from build123d import *

# Parameters (mm, degrees)
BOSS_EXTRUDE1_START         = -123.825
BOSS_EXTRUDE1_OUTLINE_R     = 6.35
BOSS_EXTRUDE1_DEPTH         = 130.175
SKETCH5_W                   = 1.4224
SKETCH5_H                   = 0.4064
F_1_4_20_TAPPED_HOLE1_D     = 5.1054
F_1_4_20_TAPPED_HOLE1_DEPTH = 16.51
F_1_4_20_TAPPED_HOLE1_TIP   = 1.533816902


# Read off the part's stored shape, not the designer's step: Boss-Extrude1
with BuildPart() as part:
    # Boss-Extrude1 outline → Boss-Extrude1 (new body)
    with BuildSketch(Plane.XY.offset(BOSS_EXTRUDE1_START)):
        Circle(BOSS_EXTRUDE1_OUTLINE_R)
    extrude(amount=BOSS_EXTRUDE1_DEPTH)

    # Sketch5 → Cut-Revolve1 (revolve, cut)
    with BuildSketch(Plane(origin=(0, 0, 0), x_dir=(0, 0, -1), z_dir=(1, 0, 0)), mode=Mode.PRIVATE) as cut_revolve1_sk:
        with Locations((-0.7112, -6.1468)):
            Rectangle(SKETCH5_W, SKETCH5_H)
    revolve(cut_revolve1_sk.sketch.rotate(Axis((0, 0, 0), (0, 0, -1)), 270), axis=Axis((0, 0, 0), (0, 0, -1)), mode=Mode.SUBTRACT)

    # 1/4-20 Tapped Hole1
    with Locations(Plane(origin=(0, 0, -123.825), x_dir=(-1, 0, 0), z_dir=(0, 0, -1))):
        with Locations((0, 0)):
            Hole(F_1_4_20_TAPPED_HOLE1_D / 2, depth=F_1_4_20_TAPPED_HOLE1_DEPTH)
            with Locations((0, 0, -(F_1_4_20_TAPPED_HOLE1_DEPTH + F_1_4_20_TAPPED_HOLE1_TIP / 2))):  # 118° drill point
                Cone(0, F_1_4_20_TAPPED_HOLE1_D / 2, F_1_4_20_TAPPED_HOLE1_TIP, mode=Mode.SUBTRACT)


solid = part.part
Design review of the part built by this model. Coordinates are the model's own, in mm. A direction names the side the tool comes from. Coordinates: 2 decimals unless noted, no trailing zeros. Order: outer loops, then holes, each group sorted by start corner. A loop starts at its lowest first (then second) coordinate and runs counter-clockwise, first axis right, second up. Notation, with made-up numbers: (84.5, 78) -> (123.5, 78) arc R24 ccw to (123.5, 117) -> close; hole circle Ø8 at (89, -8). An arc over 180 degrees is marked (long way). One line per item, written item: value.
1) We need section A-A, the plane y = -4.5. Give the boundary of the cut face in (x, z) (3 decimals).
Output values:
outline: (-4.48, -123.825) -> (4.48, -123.825) -> (4.48, 0) -> (3.883, 0) -> (3.883, 1.422) -> (4.48, 1.422) -> (4.48, 6.35) -> (-4.48, 6.35) -> (-4.48, 1.422) -> (-3.883, 1.422) -> (-3.883, 0) -> (-4.48, 0) -> close
2) We need section B-B, the plane z = -9.5. Give the boundary of the cut face in (x, y).
Output values:
outline: circle Ø12.7 at (0, 0)
3) Clearance check with flat-ended pins moving along their axes: P1, Ø4, axis at y = -3, z = -69.5, coming from the +X side; P2, Ø4, axis at x = 0, y = 0, coming from the -Z side. State where each tip first meets the part, or that it passes through.
Output values:
P1: stops at x = 6.27
P2: stops at z = -106.98
4) Draft analysis for pull direction Z (two halves, no side actions). For faces 1 (the face through (-1.38, -6.2, 3.85)), 2 (the face through (0, 0, 6.35)), 3 (the face through (5.669, -1.785, 0.701)), 4 (the face through (-0.423, 0.133, -106.048)), state which applies: +Z half, -Z half, draft (parallel to the pull), parting line (faces both ways), or undercut.
Output values:
face 1: draft
face 2: +Z half
face 3: undercut
face 4: -Z half
5) Machinability: for faces 5 (the face through (2.435, 0.767, -115.454)), 6 (the face through (3, 0, -123.825)), which of the approach directions +Z, -Z, +X, -X, +Y, -Y give a long, thin tool a straight path to every point of the face, cutting with its end or side? Answer none if there is none.
Output values:
face 5: -Z
face 6: -Z, +X, -X, +Y, -Y
6) To check wall thickness, follow probe 1 along X at (y, z) = (0, -117); probe 2 along Y at (x, z) = (-2.25, -86.5). State the ranges of each line that lie inside material, in increasing order. Write a range as [from, to].
Output values:
probe 1: x = [-6.35, -2.55], [2.55, 6.35]
probe 2: y = [-5.94, 5.94]
